```python
from build123d import *

# Parameters (mm, degrees)
SKETCH_1_R      = 2.5
EXTRUDE_1_DEPTH = 5.2
CHAMFER_1_SIZE  = 0.5


with BuildPart() as part:
    # Эскиз1 → Бобышка-Вытянуть1 (new body)
    with BuildSketch(Plane.XY):
        Polygon((0, 5.773502692), (-5, 2.886751346), (-5, -2.886751346), (0, -5.773502692), (5, -2.886751346), (5, 2.886751346), align=None)
        Circle(SKETCH_1_R, mode=Mode.SUBTRACT)
    extrude(amount=EXTRUDE_1_DEPTH)

    # Эскиз2 → Вырез-Повернуть1 (revolve, cut)
    with BuildSketch(Plane(origin=(0, 0, 0), x_dir=(0, 0, -1), z_dir=(1, 0, 0)), mode=Mode.PRIVATE) as cut_revolve_1_sk:
        Polygon((0, 5.773502692), (-0.590919555, 5.773502692), (0, 4.75), align=None)
        Polygon((-5.2, 4.75), (-5.2, 5.773502692), (-4.609080445, 5.773502692), align=None)
    revolve(cut_revolve_1_sk.sketch.rotate(Axis((0, 0, 0), (0, 0, 1)), 90), axis=Axis((0, 0, 0), (0, 0, 1)), mode=Mode.SUBTRACT)

    # Фаска1
    chamfer_1_edges = [part.edges().sort_by_distance(p)[0] for p in [
        (-2.5, 0, 0),
        (-2.5, 0, 5.2),
    ]]
    chamfer(chamfer_1_edges, length=CHAMFER_1_SIZE)


solid = part.part
```
The listing builds one solid part. Answer for the finished solid, in the listing's coordinates (mm). Round coordinates to 2 decimals unless told otherwise and drop trailing zeros. Loops run counter-clockwise (first coordinate to the right, second up) from the corner with the lowest first, then second, coordinate; pieces in that order, holes last.
Q1. Section B-B, the plane y = 0 is taken. Determine the outline of the cut face in (x, z).
Q2. Given pin 1 Ø3 at (x, z) = (0.5, 3) entering from -Y; pin 2 Ø4.5 at (x, y) = (0, 0) entering from +Z, each flat-ended and moving along its own axis, determine where each tip first touches the part or whether it passes through.
Q3. Section A-A, the plane z = 3.05 is taken. Determine the outline of the cut face in (x, y).
Q4. For a pull along X with two mould halves and no side action, classify faces 1 (the face through (-2.535, -4.31, 2.566)), 2 (the face through (-0.54, -2.44, 2.57)), 3 (the face through (2.465, -4.35, 2.566)) as released by +X, released by -X, zero draft, split by the parting line, or undercut.
Q5. Find the intervals of material crossed by line 1 (Y direction, x = 0.5, z = 3.3); line 2 (Y direction, x = 0, z = 0.35); line 3 (Y direction, x = -4.25, z = 3.5), in increasing order.
Completed:
1. outline: (-5, 0.14) - (-4.75, 0) - (-3, 0) - (-2.5, 0.5) - (-2.5, 4.7) - (-3, 5.2) - (-4.75, 5.2) - (-5, 5.06) - close; (2.5, 0.5) - (3, 0) - (4.75, 0) - (5, 0.14) - (5, 5.06) - (4.75, 5.2) - (3, 5.2) - (2.5, 4.7) - close
2. pin 1: stops at y = -5.77
2. pin 2: passes through
3. outline: (-5, -2.89) - (0, -5.77) - (5, -2.89) - (5, 2.89) - (0, 5.77) - (-5, 2.89) - close; hole circle Ø5 at (0, 0)
4. face 1: released by -X
4. face 2: undercut
4. face 3: released by +X
5. line 1: y = -5.48 to -2.45, 2.45 to 5.48
5. line 2: y = -5.36 to -2.65, 2.65 to 5.36
5. line 3: y = -3.32 to 3.32
